Check sheet for the drawn part. Datum: minimum x, y, z corner. Units: mm. Give positions to 0.01 mm unless a question says otherwise; leave off trailing zeros. Loops run counter-clockwise (first coordinate to the right, second up) from the corner with the lowest first, then second, coordinate; pieces in that order, holes last.
1. Cross-section at A-A, the plane z = 1.5. Record the cut outline in (x, y), plus the area to 3 significant figures.
2. Material ranges on L1, parallel to Y at x = 12, z = 0.85 (1 decimal); L2, parallel to Y at x = 5.5, z = 5 (1 decimal); L3, parallel to Y at x = 16.5, z = 2.25, recorded low to high.
3. Go/stop test with flat-tipped pins: pin 1 Ø4.5 at (x, y) = (12, 39) entering from -Z; pin 2 Ø3.5 at (x, y) = (9.5, 39.5) entering from +Z; pin 3 Ø4 at (x, z) = (19.5, 6.5) entering from +Y; pin 4 Ø4 at (x, z) = (5.5, 3.5) entering from +Y. Record where each tip stops, or that it passes through.
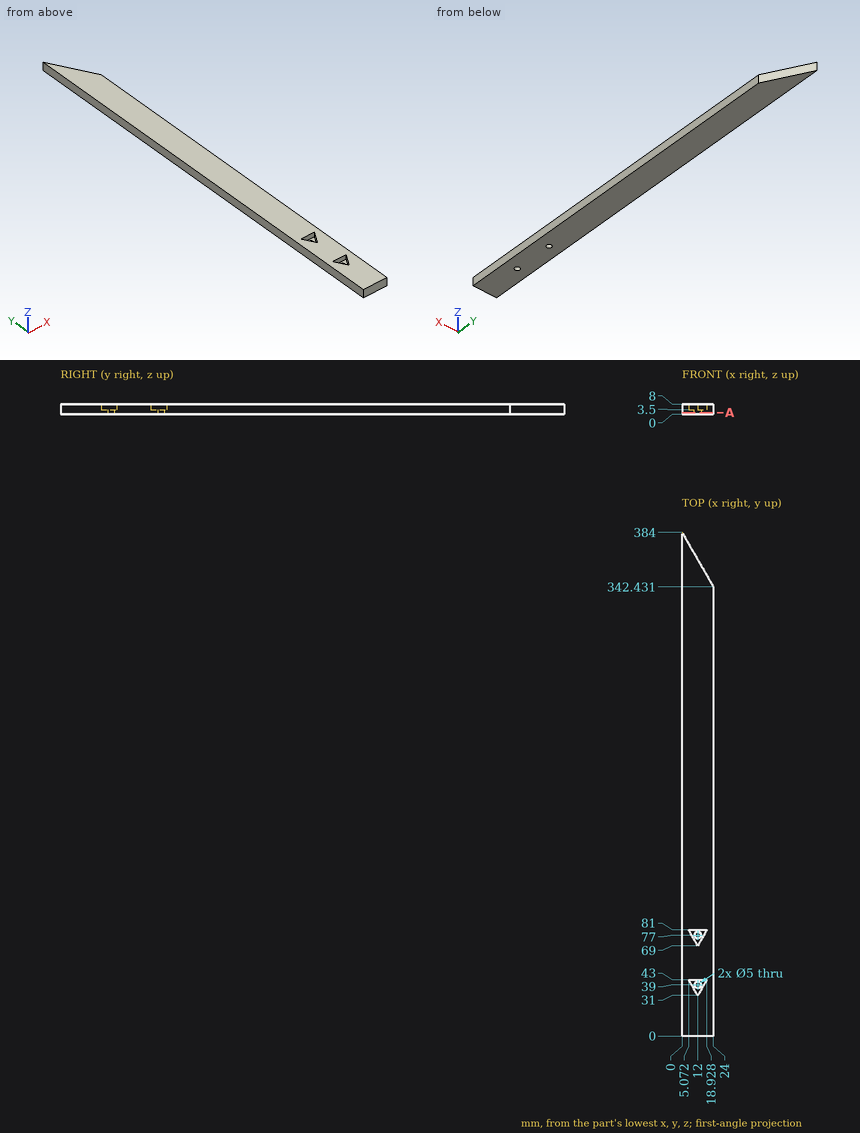
Result:
1. outline: (0, 0) - (24, 0) - (24, 342.43) - (0, 384) - close; hole circle Ø5 at (12, 39); hole circle Ø5 at (12, 77)
1. area: 8,680 mm2
2. L1: y = 0 to 36.5, 41.5 to 74.5, 79.5 to 363.2
2. L2: y = 0 to 42.3, 43 to 80.3, 81 to 374.5
2. L3: y = 0 to 355.42
3. pin 1: passes through
3. pin 2: stops at z = 3.5
3. pin 3: stops at y = 353.69
3. pin 4: stops at y = 377.94
